Input: part model. Units: mm. Frame: model coordinates. Face numbers are marked on the shaded views. A direction names the side the tool comes from. Round coordinates to 2 decimals unless told otherwise and drop trailing zeros. Loops run counter-clockwise (first coordinate to the right, second up) from the corner with the lowest first, then second, coordinate; pieces in that order, holes last.
(1) Line query: line 1 (Y direction, x = 10, z = -11.45); line 2 (Z direction, x = 11.75, y = -5.25); line 3 (Z direction, x = -0.75, y = 5). Output: solid intervals per line, ascending.
(2) Access query for the marked faces 4, 5 and 6. Directions: +Z, -Z, +X, -X, +Y, -Y. A direction counts if a zero-diameter tool reaches every point of the face in a straight line with its end or side. Return the directions, or none.
(3) First-contact query: pin 1 Ø1.5 at (x, z) = (10.5, 1.5) entering from +Y; pin 2 Ø6 at (x, z) = (-6.5, -8.5) entering from +Y; pin 3 Ø2.5 at (y, z) = (7.5, 3) entering from -X; pin 4 Ø3.5 at (x, y) = (-10, -5) entering from +Z. Flat tips, straight axial feed; report the tip coordinate or a pass-through.
(4) Cut plane A-A, the plane x = 10. Output: boundary loops of the cut face in (y, z).
(5) Cut plane B-B, the plane y = -5. Output: boundary loops of the cut face in (x, z), and give its area (3 significant figures).
(6) Cut plane C-C, the plane z = 1.25. Output: boundary loops of the cut face in (x, y), and give its area (3 significant figures).
(7) Draft query along X for the marked faces 1, 2 and 3. Return one class per face: released by +X, released by -X, zero draft, split by the parting line, or undercut.
(8) Cut plane D-D, the plane x = 0. Output: boundary loops of the cut face in (y, z).
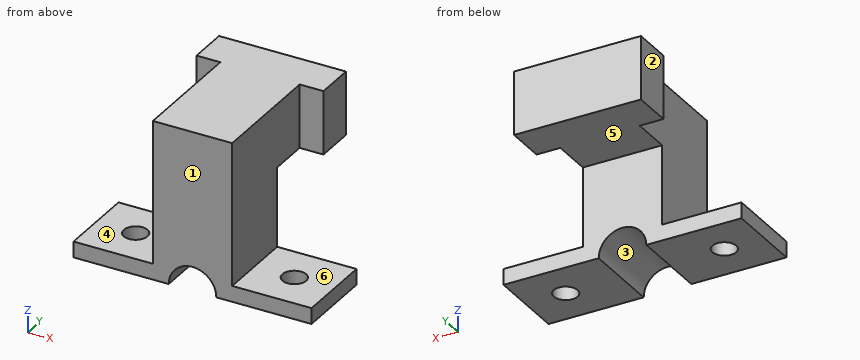
from build123d import *

# Parameters (mm, degrees)
SKETCH3_W           = 16
SKETCH3_H           = 20
BOSS_EXTRUDE1_DEPTH = 8
SKETCH4_W           = 3
SKETCH4_H           = 15
CUT_EXTRUDE1_DEPTH  = 8
SKETCH5_W           = 10
SKETCH5_H           = 10
BOSS_EXTRUDE2_DEPTH = 12
SKETCH6_R           = 3
CUT_EXTRUDE2_DEPTH  = 14
SKETCH8_W           = 2
SKETCH8_H           = 10
BOSS_EXTRUDE3_DEPTH = 10
SKETCH9_W           = 2
SKETCH9_H           = 10
BOSS_EXTRUDE4_DEPTH = 10
SKETCH10_R          = 1.5
CUT_EXTRUDE3_DEPTH  = 10


with BuildPart() as part:
    # Sketch3 → Boss-Extrude1 (new body)
    with BuildSketch(Plane.XY):
        Rectangle(SKETCH3_W, SKETCH3_H)
    extrude(amount=BOSS_EXTRUDE1_DEPTH)

    # Sketch4 → Cut-Extrude1 (cut)
    with BuildSketch(Plane.XY.offset(8)):
        with Locations((-6.5, -2.5)):
            Rectangle(SKETCH4_W, SKETCH4_H)
        with Locations((6.5, -2.5)):
            Rectangle(SKETCH4_W, SKETCH4_H)
    extrude(amount=-CUT_EXTRUDE1_DEPTH, mode=Mode.SUBTRACT)

    # Sketch5 → Boss-Extrude2 (add)
    with BuildSketch(Plane(origin=(0, 0, 0), x_dir=(-1, 0, 0), z_dir=(0, 0, -1))):
        with Locations((0, -5)):
            Rectangle(SKETCH5_W, SKETCH5_H)
    extrude(amount=BOSS_EXTRUDE2_DEPTH)

    # Sketch6 → Cut-Extrude2 (cut)
    with BuildSketch(Plane.XZ.offset(10)):
        with Locations((0, -12)):
            Circle(SKETCH6_R)
    extrude(amount=-CUT_EXTRUDE2_DEPTH, mode=Mode.SUBTRACT)

    # Sketch8 → Boss-Extrude3 (add)
    with BuildSketch(Plane(origin=(5, 0, 0), x_dir=(0, 0, -1), z_dir=(1, 0, 0))):
        with Locations((11, -5)):
            Rectangle(SKETCH8_W, SKETCH8_H)
    extrude(amount=BOSS_EXTRUDE3_DEPTH)

    # Sketch9 → Boss-Extrude4 (add)
    with BuildSketch(Plane.ZY.offset(5)):
        with Locations((-11, -5)):
            Rectangle(SKETCH9_W, SKETCH9_H)
    extrude(amount=BOSS_EXTRUDE4_DEPTH)

    # Sketch10 → Cut-Extrude3 (cut)
    with BuildSketch(Plane(origin=(0, 0, -12), x_dir=(-1, 0, 0), z_dir=(0, 0, -1))):
        with Locations((-10, -5)):
            Circle(SKETCH10_R)
        with Locations((10, -5)):
            Circle(SKETCH10_R)
    extrude(amount=-CUT_EXTRUDE3_DEPTH, mode=Mode.SUBTRACT)


solid = part.part
Reported:
1. line 1: y = -10 to -6.5, -3.5 to 0
1. line 2: z = -12 to -10
1. line 3: z = 0 to 8
2. face 4: +Z, -X, +Y, -Y
2. face 5: -Z, +X, -X, +Y
2. face 6: +Z, +X, +Y, -Y
3. pin 1: passes through
3. pin 2: stops at y = 0
3. pin 3: stops at x = -8
3. pin 4: stops at z = -10
4. outline: (-10, -12) - (-6.5, -12) - (-6.5, -10) - (-10, -10) - close; (-3.5, -12) - (0, -12) - (0, -10) - (-3.5, -10) - close
5. outline: (-15, -12) - (-11.5, -12) - (-11.5, -10) - (-15, -10) - close; (-8.5, -12) - (-3, -12) arc R3 cw to (3, -12) - (8.5, -12) - (8.5, -10) - (5, -10) - (5, 8) - (-5, 8) - (-5, -10) - (-8.5, -10) - close; (11.5, -12) - (15, -12) - (15, -10) - (11.5, -10) - close
5. area: 214 mm2
6. outline: (-8, 5) - (-5, 5) - (-5, -10) - (5, -10) - (5, 5) - (8, 5) - (8, 10) - (-8, 10) - close
6. area: 230 mm2
7. face 1: zero draft
7. face 2: released by -X
7. face 3: undercut
8. outline: (-10, -9) - (0, -9) - (0, 0) - (10, 0) - (10, 8) - (-10, 8) - close
